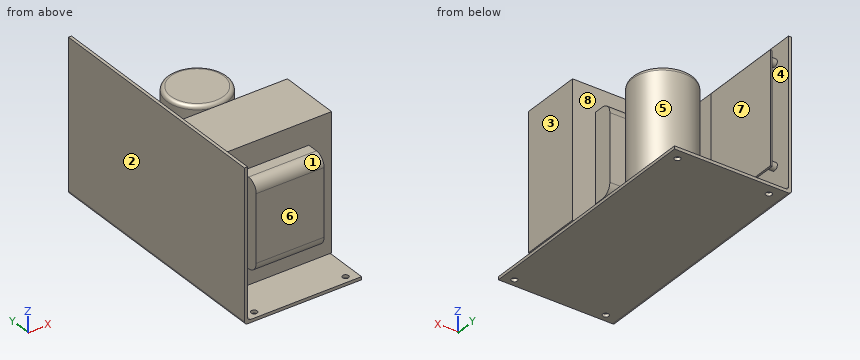
```python
from build123d import *

# Parameters (mm, degrees)
F1_DEPTH      = 205.74
F3_D          = 5.08
F4_R          = 2.54
F5_W          = 51.562
F5_H          = 114.3
F6_DEPTH      = 95.504
F7_W          = 57.15
F7_H          = 74.168
F8_DEPTH      = 17.78
F8_DEPTH_BACK = 68.58
F9_R          = 25.4
F10_DEPTH     = 84.328
F11_R         = 3.175
F12_R         = 8.89
F13_R         = 3.175
F14_DEPTH     = 6.35
F15_W         = 69.342
F15_H         = 93.98
F16_DEPTH     = 1.524


with BuildPart() as f1:
    # F0 (on Front) → F1 (new body)
    with BuildSketch(Plane.XZ):
        Polygon((0, 127), (0, 0), (98.552, 0), (98.552, 2.54), (2.54, 2.54), (2.54, 127), align=None)
    extrude(amount=F1_DEPTH)

    # F3 (through all)
    with Locations(Plane(origin=(0, 0, 0), x_dir=(1, 0, 0), z_dir=(0, 0, -1))):
        with Locations((12.7, 199.39), (89.662, 199.39), (89.662, 8.89), (12.7, 8.89)):
            Hole(F3_D / 2)

    # F4
    f4_edges = [f1.edges().sort_by_distance(p)[0] for p in [
        (0, -102.87, 0),
        (2.54, -102.87, 2.54),
    ]]
    fillet(f4_edges, radius=F4_R)

    # F5 (on face) → F6 (join)
    with BuildSketch(Plane.YZ.offset(2.54)):
        with Locations((-145.669, 61.468)):
            Rectangle(F5_W, F5_H)
    extrude(amount=F6_DEPTH)

    # F7 (on face) → F8 (join, two sides)
    with BuildSketch(Plane.XZ.offset(171.45)) as f8_sk:
        with Locations((50.292, 61.468)):
            Rectangle(F7_W, F7_H)
    extrude(amount=F8_DEPTH)
    extrude(f8_sk.sketch, amount=-F8_DEPTH_BACK)

    # F9 (on face) → F10 (join)
    with BuildSketch(Plane.XY.offset(2.54)):
        with Locations((71.882, -50.8)):
            Circle(F9_R)
    extrude(amount=F10_DEPTH)

    # F11
    f11_edges = [f1.edges().sort_by_distance(p)[0] for p in [
        (46.482, -50.8, 86.868),
    ]]
    fillet(f11_edges, radius=F11_R)

    # F12
    f12_edges = [f1.edges().sort_by_distance(p)[0] for p in [
        (50.292, -189.23, 98.552),
        (50.292, -189.23, 24.384),
        (50.292, -102.87, 98.552),
        (50.292, -102.87, 24.384),
    ]]
    fillet(f12_edges, radius=F12_R)

    # F13 (on face) → F14 (join)
    with BuildSketch(Plane.YZ.offset(2.54)):
        with Locations((-73.914, 113.284)):
            Circle(F13_R)
        with Locations((-16.256, 113.284)):
            Circle(F13_R)
        with Locations((-16.256, 29.464)):
            Circle(F13_R)
        with Locations((-73.914, 29.464)):
            Circle(F13_R)
    extrude(amount=F14_DEPTH)

    # F15 (on face) → F16 (join)
    with BuildSketch(Plane.YZ.offset(8.89)):
        with Locations((-45.085, 71.374)):
            Rectangle(F15_W, F15_H)
    extrude(amount=F16_DEPTH)


solid = f1.part
```
The listing builds one solid part. Answer for the finished solid, in the listing's coordinates (mm). Face numbers are marked on the shaded views. A direction names the side the tool comes from. Give positions to 0.01 mm unless a question says otherwise; leave off trailing zeros. Order: outer loops, then holes, each group sorted by start corner. A loop starts at its lowest first (then second) coordinate and runs counter-clockwise, first axis right, second up. Notation, with made-up numbers: (19, 55.25) - (62, 55.25) arc R18 cw to (62, 61.25) - close; hole circle Ø8 at (-21.75, 40.25). An arc over 180 degrees is marked (long way). Answer in a Markdown table with one row per item. Add a question column.
Q1. Find the intervals of material crossed by line 1 along X through (y, z) = (-8, 1); line 2 along Z through (x, y) = (14.5, -121); line 3 along X through (y, z) = (-8.89, 0.9), in increasing order. Write a range as [from, to].
Q2. Given P1, Ø7, axis at x = 42.5, y = -177, coming from the +Z side; P2, Ø12, axis at y = -173.5, z = 80, coming from the +X side; P3, Ø3, axis at x = 25.5, y = -33, coming from the +Z side, each flat-ended and moving along its own axis, determine where each tip first touches the part or whether it passes through.
Q3. The part is cut by section B-B (z = 46.5). Determine the outline of the cut face in (x, y), then the cut area to 3 significant figures.
Q4. The part is cut by section D-D (y = -50.8). Determine the outline of the cut face in (x, z) (3 decimals).
Q5. For a pull along X with two mould halves and no side action, classify the marked faces 1, 2, 3 and 4 as released by +X, released by -X, zero draft, split by the parting line, or undercut.
Q6. The part is cut by section C-C (y = -199.39). Determine the outline of the cut face in (x, z), then the cut area to 3 significant figures.
Q7. The part is cut by section A-A (x = 32). Determine the outline of the cut face in (y, z).
Q8. Which of the six approach directions +Z, -Z, +X, -X, +Y, -Y give full straight-line access (tool end or side, diameter ignored) to the marked faces 5, 6, 7 and 8?
Determined:
| question | item | result |
|---|---|---|
| 1 | line 1 | x = [0.52, 10.32], [15.08, 87.28], [92.04, 98.55] |
| 1 | line 2 | z = [0, 2.54], [4.32, 118.62] |
| 1 | line 3 | x = [0.6, 10.16], [15.24, 87.12], [92.2, 98.55] |
| 2 | P1 | stops at z = 98.55 |
| 2 | P2 | stops at x = 98.04 |
| 2 | P3 | stops at z = 2.54 |
| 3 | outline | (0, -205.74) - (2.54, -205.74) - (2.54, -171.45) - (21.72, -171.45) - (21.72, -189.23) - (78.87, -189.23) - (78.87, -171.45) - (98.04, -171.45) - (98.04, -119.89) - (78.87, -119.89) - (78.87, -102.87) - (21.72, -102.87) - (21.72, -119.89) - (2.54, -119.89) - (2.54, 0) - (0, 0) - close; (8.89, -79.76) - (10.41, -79.76) - (10.41, -10.41) - (8.89, -10.41) - close; circle Ø50.8 at (71.88, -50.8) |
| 3 | area | 9,570 mm² |
| 4 | outline | (0, 2.54) arc R2.54 ccw to (2.54, 0) - (98.552, 0) - (98.552, 2.54) - (97.282, 2.54) - (97.282, 83.693) arc R3.175 ccw to (94.107, 86.868) - (49.657, 86.868) arc R3.175 ccw to (46.482, 83.693) - (46.482, 2.54) - (5.08, 2.54) arc R2.54 cw to (2.54, 5.08) - (2.54, 127) - (0, 127) - close; (8.89, 24.384) - (10.414, 24.384) - (10.414, 118.364) - (8.89, 118.364) - close |
| 5 | face 1 | zero draft |
| 5 | face 2 | released by -X |
| 5 | face 3 | released by +X |
| 5 | face 4 | undercut |
| 6 | outline | (0, 2.54) arc R2.54 ccw to (2.54, 0) - (10.16, 0) - (10.16, 2.54) - (5.08, 2.54) arc R2.54 cw to (2.54, 5.08) - (2.54, 127) - (0, 127) - close; (15.24, 0) - (87.12, 0) - (87.12, 2.54) - (15.24, 2.54) - close; (92.2, 0) - (98.55, 0) - (98.55, 2.54) - (92.2, 2.54) - close |
| 6 | area | 541 mm² |
| 7 | outline | (-205.74, 0) - (0, 0) - (0, 2.54) - (-205.74, 2.54) - close; (-189.23, 33.27) arc R8.89 ccw to (-180.34, 24.38) - (-171.45, 24.38) - (-171.45, 4.32) - (-119.89, 4.32) - (-119.89, 24.38) - (-111.76, 24.38) arc R8.89 ccw to (-102.87, 33.27) - (-102.87, 89.66) arc R8.89 ccw to (-111.76, 98.55) - (-119.89, 98.55) - (-119.89, 118.62) - (-171.45, 118.62) - (-171.45, 98.55) - (-180.34, 98.55) arc R8.89 ccw to (-189.23, 89.66) - close |
| 8 | face 5 | +Z |
| 8 | face 6 | +Z, +X, -Y |
| 8 | face 7 | +Z, +Y |
| 8 | face 8 | none |
